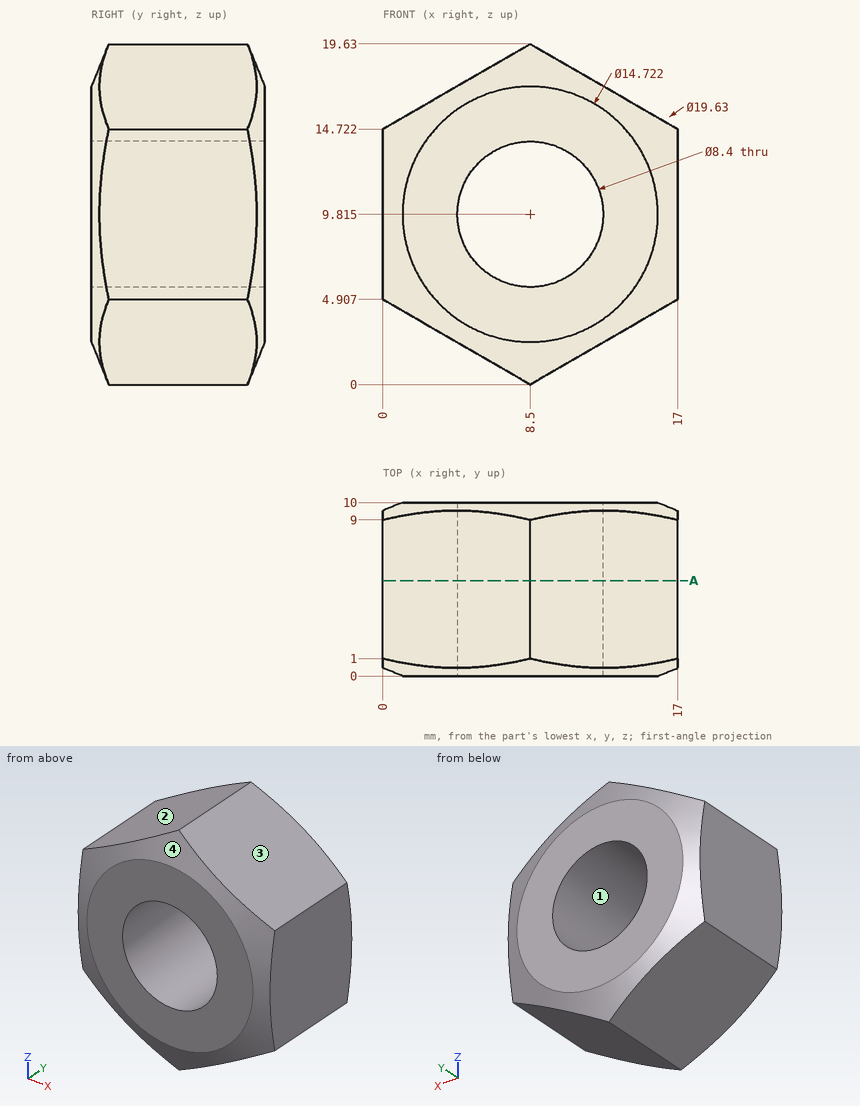
Geometry: see drawing. Coordinates: mm, zero at the bounding-box minimum. Give positions to 0.01 mm unless a question says otherwise; leave off trailing zeros. Order: outer loops, then holes, each group sorted by start corner. A loop starts at its lowest first (then second) coordinate and runs counter-clockwise, first axis right, second up. Notation, with made-up numbers: (29, 45) - (79, 45) arc R12 cw to (79, 52) - close; hole circle Ø1 at (35, -8.5). An arc over 180 degrees is marked (long way). One line per item, written item: value.
1. Draft query along X for the marked faces 1, 2, 3 and 4. Return one class per face: released by +X, released by -X, zero draft, split by the parting line, or undercut.
Determined:
face 1: undercut
face 2: released by -X
face 3: released by +X
face 4: split by the parting line
2. Cut plane A-A, the plane y = 5.5. Output: boundary loops of the cut face in (x, z) (1 decimal), and give its area (3 significant figures).
Determined:
outline: (0, 4.9) - (8.5, 0) - (17, 4.9) - (17, 14.7) - (8.5, 19.6) - (0, 14.7) - close; hole circle Ø8.4 at (8.5, 9.8)
area: 195 mm2
3. Line query: probe 1 along X at (y, z) = (5, 9.75); probe 2 along Z at (x, y) = (11.5, 3.5) (1 decimal); probe 3 along Z at (x, y) = (11.25, 2). Output: solid intervals per line, ascending.
Determined:
probe 1: 0 to 4.3, 12.7 to 17
probe 2: 1.7 to 6.9, 12.8 to 17.9
probe 3: 1.59 to 6.64, 12.99 to 18.04
